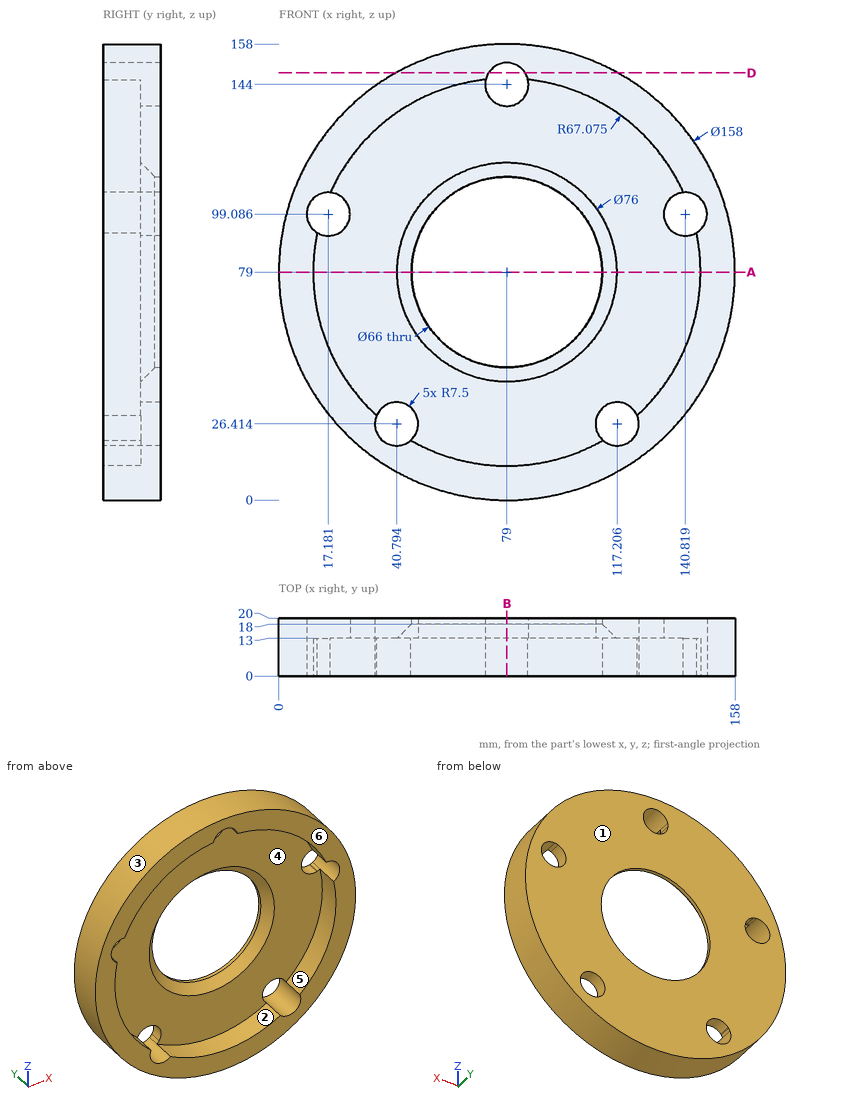
Part print with two shaded views. Sizes in mm from the minimum x, y, z corner. A direction names the side the tool comes from. Coordinates: 2 decimals unless noted, no trailing zeros. Write each loop counter-clockwise with the first axis right and the second up, starting at its lowest first coordinate (ties: lowest second). Pieces come first, ordered by that corner, then holes.
(1) Pin check, flat tips, straight feed: pin 1 Ø4 at (y, z) = (5.5, 114.5) entering from +X (1 decimal); pin 2 Ø2 at (x, z) = (34.5, 45.5) entering from -Y; pin 3 Ø10 at (y, z) = (16.5, 132.5) entering from +X. Stop position of each tip, or through.
(2) Cut at D-D on z = 148. List the corners of the cut face in (x, y).
(3) Cut at B-B on x = 79. List the corners of the cut face in (y, z) (1 decimal).
(4) Mould opens along Z. For the marked faces 1, 2, 3 and 4 say: pulls with the +Z half, pulls with the -Z half, needs draft (parallel to the pull), parting line crosses it, or undercut.
(5) Cut at A-A on z = 79. List the corners of the cut face in (x, y) (1 decimal).
(6) Drill centre lines: line 1 (Z direction, x = 79, y = 19.45); line 2 (Y direction, x = 30, z = 61); line 3 (X direction, y = 10.75, z = 32) (1 decimal). Where is each one in solid material? Low to high.
(7) 3-axis set-ups, long thin cutter, end or side, ignore diameter. For the marked faces 5 and 6: which of +Z, -Z, +X, -X, +Y, -Y reach the whole face in a straight line?
Working result:
1. pin 1: stops at x = 150.5
1. pin 2: stops at y = 13
1. pin 3: stops at x = 141.36
2. outline: (40.53, 0) - (72.66, 0) - (72.66, 20) - (40.53, 20) - close; (85.34, 0) - (117.47, 0) - (117.47, 20) - (85.34, 20) - close
3. outline: (0, 0) - (20, 0) - (20, 46) - (18, 46) - (13, 41) - (13, 11.9) - (0, 11.9) - close; (0, 151.5) - (20, 151.5) - (20, 158) - (0, 158) - close; (13, 117) - (18, 112) - (20, 112) - (20, 136.5) - (13, 136.5) - close
4. face 1: needs draft
4. face 2: undercut
4. face 3: parting line crosses it
4. face 4: undercut
5. outline: (0, 0) - (11.9, 0) - (11.9, 13) - (41, 13) - (46, 18) - (46, 20) - (0, 20) - close; (112, 18) - (117, 13) - (146.1, 13) - (146.1, 0) - (158, 0) - (158, 20) - (112, 20) - close
6. line 1: z = 0 to 46, 112 to 136.5, 151.5 to 158
6. line 2: y = 13 to 20
6. line 3: x = 15.5 to 31.1, 126.9 to 142.5
7. face 5: -Y
7. face 6: +Z, -Z, +X, -X, -Y
